Read the model definition and answer for the solid it produces. Units are mm, in the model's axes. A direction names the side the tool comes from. Give positions to 0.01 mm unless a question says otherwise; leave off trailing zeros. Loops run counter-clockwise (first coordinate to the right, second up) from the corner with the lowest first, then second, coordinate; pieces in that order, holes last. Notation, with made-up numbers: (-24, 74.5) - (-8, 74.5) arc R20 ccw to (-8, 103.5) - close; hole circle Ø9 at (-15.5, 44). An arc over 180 degrees is marked (long way). Use a Markdown table: item, result. Add a question column.
Item 1: For a pull along X with two mould halves and no side action, classify faces 3 (the face through (-78.265, 3.768, -4.306)), 4 (the face through (-85, 2, -3)), 5 (the face through (-42, 0, -3)) as +X half, -X half, draft (parallel to the pull), parting line (faces both ways), or undercut.
Item 2: A cutting plane is placed at C-C (x = -8). Determine the outline of the cut face in (y, z).
Item 3: A cutting plane is placed at A-A (z = -3.5). Determine the outline of the cut face in (x, y).
Item 4: A cutting plane is placed at B-B (y = 3.7). Determine the outline of the cut face in (x, z).
Item 5: Consider probe 1 along X at (y, z) = (4.1, -3.5); probe 2 along X at (y, z) = (0.95, -3.5); probe 3 along Z at (x, y) = (-8, 0.7). Determine where each line is inside the solid, lowest interval first. Write a range as [from, to].
Item 6: Each of these flat-tipped pins is pushed along its axis until it touches: P1, Ø1, axis at x = -69, y = 2, coming from the +Z side; P2, Ø2.5, axis at x = -77, z = -3.5, coming from the -Y side; P3, Ø3, axis at x = -77, z = -4, coming from the -Y side. Where does it stop, or does it pass through?
Item 7: Which of the six approach directions +Z, -Z, +X, -X, +Y, -Y give full straight-line access (tool end or side, diameter ignored) to faces 1 (the face through (-8.1, 1.3, -0.5)), 2 (the face through (-42, 2, 0))?
Autodesk Inventor part; units mm, degrees
ref_plane "YZ Plane" through (0, 0, 0) normal (1, 0, 0) x (0, 1, 0)
ref_plane "XZ Plane" through (0, 0, 0) normal (0, 1, 0) x (-1, 0, 0)
ref_plane "XY Plane" through (0, 0, 0) normal (0, 0, 1) x (1, 0, 0)
sketch "Sketch1" plane through (0, 0, 0) normal (0, 1, 0) x (-1, 0, 0)
  line L0 (0, 0) -> (85, 0)
  line L1 (85, 0) -> (85, -7)
  line L2 (85, -7) -> (0, -7)
  line L3 (0, -7) -> (0, 0)
  line L4 (42.5, 3) -> (42.5, -16) construction
  line L5 (45, -3.5) -> (39, -3.5) construction
  point P0 (77, -3.5)
  point P1 (8, -3.5)
  dimension "d0" = 85
  dimension "d1" = 7
  dimension "d2" = 69
  dimension "d12" = 3.5
extrude "Extrusion1" add sketch "Sketch1" along normal blind 5
hole "Hole1" at (-77, 0, -3.5) at (-8, 0, -3.5) direction (0, 1, 0) diameter 3 end through all counterbore diameter 6 counterbore depth 2.5
properties part number "Rail" material "Wood (Birch)"
Geometry says:
| question | item | result |
|---|---|---|
| 1 | face 3 | undercut |
| 1 | face 4 | -X half |
| 1 | face 5 | draft |
| 2 | outline | (0, -7) - (5, -7) - (5, -5) - (2.5, -5) - (2.5, -6.5) - (0, -6.5) - close; (0, -0.5) - (2.5, -0.5) - (2.5, -2) - (5, -2) - (5, 0) - (0, 0) - close |
| 3 | outline | (-85, 0) - (-80, 0) - (-80, 2.5) - (-78.5, 2.5) - (-78.5, 5) - (-85, 5) - close; (-75.5, 2.5) - (-74, 2.5) - (-74, 0) - (-11, 0) - (-11, 2.5) - (-9.5, 2.5) - (-9.5, 5) - (-75.5, 5) - close; (-6.5, 2.5) - (-5, 2.5) - (-5, 0) - (0, 0) - (0, 5) - (-6.5, 5) - close |
| 4 | outline | (-85, -7) - (0, -7) - (0, 0) - (-85, 0) - close; hole circle Ø3 at (-77, -3.5); hole circle Ø3 at (-8, -3.5) |
| 5 | probe 1 | [-85, -78.5], [-75.5, -9.5], [-6.5, 0] |
| 5 | probe 2 | [-85, -80], [-74, -11], [-5, 0] |
| 5 | probe 3 | [-7, -6.5], [-0.5, 0] |
| 6 | P1 | z = 0 |
| 6 | P2 | through |
| 6 | P3 | y = 2.5 |
| 7 | face 1 | -Y |
| 7 | face 2 | +Z, +X, -X, +Y, -Y |
